For this review, take the finished solid that the model builds, in its own axes (mm). Face numbers are marked on the shaded views. A direction names the side the tool comes from. Round coordinates to 2 decimals unless told otherwise and drop trailing zeros. Write each loop counter-clockwise with the first axis right and the second up, starting at its lowest first coordinate (ties: lowest second). Pieces come first, ordered by that corner, then holes. Notation, with made-up numbers: M 57,19.25 L 88,19.25 A12 ccw 88,27.25 Z; hole C 40,46.25 d11. An arc over 180 degrees is marked long. One line per question, with ' | ' between items.
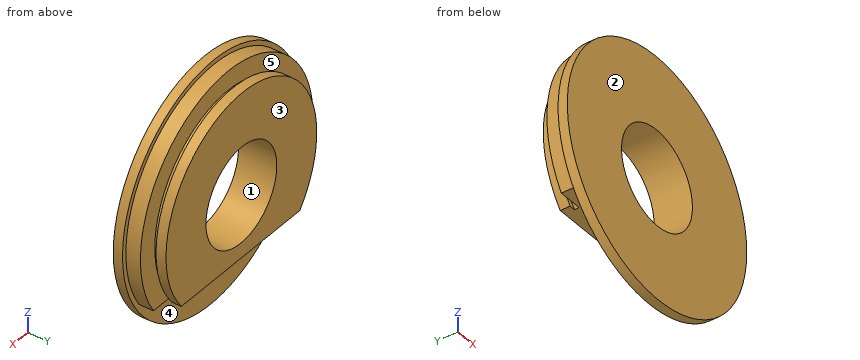
```python
from build123d import *

# Parameters (mm, degrees)
CUT_EXTRUDE1_DEPTH = 9.5


with BuildPart() as part:
    # Sketch1 → Revolve1 (revolve)
    with BuildSketch(Plane.XY):
        Polygon((15.802589648, 0), (40, 0), (40, 3), (38.5, 3), (38.5, 7.75), (32.113475553, 7.75), (32.113475553, 9.25), (33.613475553, 9.25), (33.613475553, 12.5), (15.802589648, 12.5), align=None)
    revolve(axis=Axis((0, 0, 0), (0, 1, 0)))

    # Sketch2 → Cut-Extrude1 (cut)
    with BuildSketch(Plane(origin=(0, 12.5, 0), x_dir=(1, 0, 0), z_dir=(0, 1, 0))):
        with BuildLine():
            Line((-32.06723123, 21.305930659), (32.696608404, 20.326873809))
            ThreePointArc((32.696608404, 20.326873809), (0.581951017, 38.495601476), (-32.06723123, 21.305930659))
        make_face()
    extrude(amount=-CUT_EXTRUDE1_DEPTH, mode=Mode.SUBTRACT)


solid = part.part
```
Item 1: To check wall thickness, follow line 1 along X through (y, z) = (5.25, 0); line 2 along Y through (x, z) = (-25.5, 23); line 3 along Z through (x, y) = (0, 4.75). State the ranges of each line that lie inside material, in increasing order. Write a range as from..to.
Results:
line 1: -38.5..-15.8, 15.8..38.5 | line 2: 0..7.75 | line 3: -20.82..-15.8, 15.8..38.5
Item 2: Take a section at A-A (z = 0). Write out the cut boundary in (x, y).
Results:
outline: M -40,0 L -15.8,0 L -15.8,12.5 L -33.61,12.5 L -33.61,9.25 L -32.11,9.25 L -32.11,7.75 L -38.5,7.75 L -38.5,3 L -40,3 Z; M 15.8,0 L 40,0 L 40,3 L 38.5,3 L 38.5,7.75 L 32.11,7.75 L 32.11,9.25 L 33.61,9.25 L 33.61,12.5 L 15.8,12.5 Z
Item 3: Insertion check: pin 1 Ø1 at (x, y) = (5.5, 8) entering from -Z; pin 2 Ø5 at (x, z) = (-24, 27) entering from -Y; pin 3 Ø6 at (x, y) = (-18, 5) entering from +Z; pin 4 Ø4 at (x, z) = (1.5, -23) entering from +Y. Each pin has a flat end and moves straight along its axis. Give the tip position at first contact, or say it passes through.
Results:
pin 1: z = -20.75 | pin 2: y = 0 | pin 3: z = 36.76 | pin 4: y = 3
Item 4: Take a section at B-B (x = -14). Write out the cut boundary in (y, z).
Results:
outline: M 0,-37.47 L 3,-37.47 L 3,-21.03 L 12.5,-21.03 L 12.5,-7.33 L 0,-7.33 Z; M 0,7.33 L 12.5,7.33 L 12.5,30.56 L 9.25,30.56 L 9.25,28.9 L 7.75,28.9 L 7.75,35.86 L 3,35.86 L 3,37.47 L 0,37.47 Z
Item 5: Mouldability with a two-part tool opening along Z and no side actions: class the marked faces 1 and 2 as +Z half, -Z half, draft (parallel to the pull), parting line (faces both ways), or undercut.
Results:
face 1: undercut | face 2: draft
Item 6: Machinability: for the marked faces 3, 4 and 5, which of the approach directions +Z, -Z, +X, -X, +Y, -Y give a long, thin tool a straight path to every point of the face, cutting with its end or side? Answer none if there is none.
Results:
face 3: +Z, -Z, +X, -X, +Y | face 4: +Y | face 5: none
Item 7: Take a section at D-D (z = 17). Write out the cut boundary in (x, y), then the cut area to 3 significant figures.
Results:
outline: M -36.21,0 L 36.21,0 L 36.21,3 L 34.54,3 L 34.54,7.75 L 27.24,7.75 L 27.24,9.25 L 29,9.25 L 29,12.5 L -29,12.5 L -29,9.25 L -27.24,9.25 L -27.24,7.75 L -34.54,7.75 L -34.54,3 L -36.21,3 Z | area: 816 mm2
Item 8: Take a section at C-C (y = 2). Write out the cut boundary in (x, z), then the cut area to 3 significant figures.
Results:
outline: C 0,0 d80; hole C 0,0 d31.61 | area: 4,240 mm2
